Design review of the part built by this model. Coordinates are the model's own, in mm. A direction names the side the tool comes from. Coordinates: 2 decimals unless noted, no trailing zeros. Write each loop counter-clockwise with the first axis right and the second up, starting at its lowest first coordinate (ties: lowest second). Pieces come first, ordered by that corner, then holes. Notation, with made-up numbers: (-35.75, 60.5) - (-19.75, 60.5) arc R13 cw to (-19.75, 83.5) - close; hole circle Ø1 at (9, 22.5). An arc over 180 degrees is marked (long way). Use a Markdown table: item, result.
from build123d import *

# Parameters (mm, degrees)
SKETCH1_R           = 4
SKETCH1_R_2         = 1.5
BOSS_EXTRUDE1_DEPTH = 2.75
SKETCH2_R           = 1.5
BOSS_EXTRUDE2_DEPTH = 2.7
CUT_EXTRUDE1_DEPTH  = 0.55
FILLET1_R           = 3
CHAMFER1_SIZE       = 1.3
CUT_EXTRUDE3_DEPTH  = 2.7


with BuildPart() as part:
    # Sketch1 → Boss-Extrude1 (new body)
    with BuildSketch(Plane(origin=(0, 0, 0), x_dir=(1, 0, 0), z_dir=(0, 1, 0))):
        with BuildLine():
            Line((4.884776311, 13.5), (-55, 13.5))
            Line((-55, 13.5), (-55, 7.5))
            Line((-55, 7.5), (-42.906998157, 7.5))
            Line((-42.906998157, 7.5), (-26.5, -13.5))
            Line((-26.5, -13.5), (-24, -13.5))
            ThreePointArc((-24, -13.5), (-13, -11.5), (-2, -13.5))
            Line((-2, -13.5), (7.5, -13.5))
            Line((7.5, -13.5), (10.675426481, -8))
            Line((10.675426481, -8), (8, -8))
            Line((8, -8), (8, 10.384776311))
            Line((8, 10.384776311), (4.884776311, 13.5))
        make_face()
        Circle(SKETCH1_R, mode=Mode.SUBTRACT)
        with Locations((-36, 8)):
            Circle(SKETCH1_R_2, mode=Mode.SUBTRACT)
    extrude(amount=BOSS_EXTRUDE1_DEPTH)

    # Sketch2 → Boss-Extrude2 (add)
    with BuildSketch(Plane(origin=(0, 2.75, 0), x_dir=(1, 0, 0), z_dir=(0, 1, 0))):
        Polygon((-39.781855651, 3.5), (-13.523502692, 3.5), (-7.75, 13.5), (-55, 13.5), (-55, 7.5), (-42.906998157, 7.5), align=None)
        with Locations((-36, 8)):
            Circle(SKETCH2_R, mode=Mode.SUBTRACT)
    extrude(amount=BOSS_EXTRUDE2_DEPTH)

    # Sketch3 → Cut-Extrude1 (cut)
    with BuildSketch(Plane.XZ):
        Polygon((-23, -10.5), (-55, -10.5), (-55, 9.5), (-7.37428747, 9.5), align=None)
    extrude(amount=-CUT_EXTRUDE1_DEPTH, mode=Mode.SUBTRACT)

    # Fillet1
    fillet1_edges = [part.edges().sort_by_distance(p)[0] for p in [
        (-55, 3, -7.5),
    ]]
    fillet(fillet1_edges, radius=FILLET1_R)

    # Chamfer1
    chamfer1_edges = [part.edges().sort_by_distance(p)[0] for p in [
        (-31.375, 5.45, -13.5),
    ]]
    chamfer(chamfer1_edges, length=CHAMFER1_SIZE)

    # Mirror1: part across plane


with BuildPart() as part_1:
    add(part.part)
    add(part.part.mirror(Plane.ZX))

    # Sketch6 → Cut-Extrude3 (cut)
    with BuildSketch(Plane.XZ.offset(5.45)):
        Polygon((-32.218144349, -3.5), (-28.311716217, -8.5), (-10.636751346, -8.5), (-13.523502692, -3.5), align=None)
    extrude(amount=-CUT_EXTRUDE3_DEPTH, mode=Mode.SUBTRACT)

    # Sketch7 → Cut-Revolve1 (revolve, cut)
    with BuildSketch(Plane(origin=(0, 0, 0), x_dir=(0.999390827, 0, 0.034899497), z_dir=(-0.034899497, 0, 0.999390827))):
        with BuildLine():
            Line((-10, -2.75), (-10, -1.75))
            ThreePointArc((-10, -1.75), (-11.118033989, -2.013932023), (-12, -2.75))
            Line((-12, -2.75), (-10, -2.75))
        make_face()
    revolve(axis=Axis((-9.99390827, -10.952082058, -0.348994967), (0, 1, 0)), mode=Mode.SUBTRACT)


solid = part_1.part
(1) Machinability: for faces 4 (the flat face through (-15.08, 0.01, -0.36)), 5 (the flat face through (-9, -2.75, 3)), 6 (the flat face through (-36, -4, -3.5)), which of the approach directions +Z, -Z, +X, -X, +Y, -Y give a long, thin tool a straight path to every point of the face, cutting with its end or side? Answer none if there is none.
Determined:
| item | result |
|---|---|
| face 4 | -X |
| face 5 | +Z, +X, -Y |
| face 6 | +Z, +X, -X, -Y |
(2) Take a section at B-B on y = -3.5. Write out the cut boundary in (x, z), and give its area (3 significant figures).
Determined:
| item | result |
|---|---|
| outline | (-55, -13.5) - (-7.75, -13.5) - (-10.64, -8.5) - (-28.31, -8.5) - (-32.22, -3.5) - (-39.78, -3.5) - (-42.91, -7.5) - (-52, -7.5) arc R3 ccw to (-55, -10.5) - close; hole circle Ø3 at (-36, -8) |
| area | 289 mm2 |
(3) For L1, parallel to Y at x = -51, z = -8; L2, parallel to Z at x = -36, y = 3.9; L3, parallel to Y at x = -21, z = 0, list the stretches that pass through material, from the lowest coordinate up. Write a range as from..to.
Determined:
| item | result |
|---|---|
| L1 | -5.45..-0.55, 0.55..5.45 |
| L2 | -13.5..-9.5, -6.5..-3.5 |
| L3 | -2.75..-0.55, 0.55..2.75 |
(4) Take a section at C-C on x = -36. Write out the cut boundary in (y, z).
Determined:
| item | result |
|---|---|
| outline | (-5.45, -12.2) - (-4.15, -13.5) - (4.15, -13.5) - (5.45, -12.2) - (5.45, -9.5) - (0.55, -9.5) - (0.55, -10.5) - (-0.55, -10.5) - (-0.55, -9.5) - (-5.45, -9.5) - close; (-5.45, -6.5) - (-0.55, -6.5) - (-0.55, 1.34) - (-2.75, 1.34) - (-2.75, -3.5) - (-5.45, -3.5) - close; (0.55, -6.5) - (5.45, -6.5) - (5.45, -3.5) - (2.75, -3.5) - (2.75, 1.34) - (0.55, 1.34) - close |
(5) Take a section at D-D on z = 6. Write out the cut boundary in (x, y), and give its area (3 significant figures).
Determined:
| item | result |
|---|---|
| outline | (-32.36, -2.75) - (8, -2.75) - (8, 2.75) - (-32.36, 2.75) - (-32.36, 0.55) - (-10.11, 0.55) - (-10.11, -0.55) - (-32.36, -0.55) - close |
| area | 198 mm2 |
(6) Draft analysis for pull direction Z (two halves, no side actions). For faces 1 (the cylindrical face through (-37.2, 3, -7.1)), 2 (the flat face through (-10.677, 4.081, -8.43)), 3 (the flat face through (8, 0, -1)), state which applies: +Z half, -Z half, draft (parallel to the pull), parting line (faces both ways), or undercut.
Determined:
| item | result |
|---|---|
| face 1 | undercut |
| face 2 | +Z half |
| face 3 | draft |
(7) Take a section at A-A on x = 0. Write out the cut boundary in (y, z).
Determined:
| item | result |
|---|---|
| outline | (-2.75, -13.5) - (2.75, -13.5) - (2.75, -4) - (-2.75, -4) - close; (-2.75, 4) - (2.75, 4) - (2.75, 13.5) - (-2.75, 13.5) - close |
(8) For pin 1 (1 mm diameter, centred on x = -2.5, z = -4.5, fed in from +Y); pin 2 (3 mm diameter, centred on x = -4, z = -6.5, fed in from -Y); pin 3 (3 mm diameter, centred on y = -1.5, z = -9.5, fed in from -X); pin 4 (2.5 mm diameter, centred on x = -48, y = -3.5, fed in from +Z), all flat-tipped, find the tip position at first contact; note any pin that passes through.
Determined:
| item | result |
|---|---|
| pin 1 | y = 2.75 |
| pin 2 | y = -2.75 |
| pin 3 | x = -55 |
| pin 4 | z = -7.5 |
